Can you work these out from the model? Positions are in its coordinate system, mm. Face numbers are marked on the shaded views. A direction names the side the tool comes from. Round coordinates to 2 decimals unless told otherwise and drop trailing zeros. Write each loop counter-clockwise with the first axis right and the second up, starting at its lowest first coordinate (ties: lowest second). Pieces come first, ordered by that corner, then holes. Notation, with made-up numbers: M 35,56.25 L 73,56.25 A16 ccw 73,84.25 Z; hole C 0.5,76.5 d6. An arc over 180 degrees is marked long. Answer as a JSON object with one key per item and string values. Group by question number.
1) Suppose I cut it at D-D, the plane x = 7. Write out the boundary of the cut face in (y, z), and give its area (3 significant figures).
2) Please list where these lines run through material, in increasing order: L1, parallel to X at y = -2.75, z = 232; L2, parallel to Z at x = 0, y = -4; L3, parallel to Z at x = 11, y = -3.5. Write a range as [from, to].
3) Suppose I cut it at B-B, the plane z = 46.5. Write out the boundary of the cut face in (x, y).
4) Suppose I cut it at C-C, the plane x = -6. Write out the boundary of the cut face in (y, z).
5) Suppose I cut it at A-A, the plane y = 0. Write out the boundary of the cut face in (x, z), and give its area (3 significant figures).
6) I'm going to push flat-ended pins straight in: pin 1 Ø3 at (x, z) = (4.5, 138) entering from +Y; pin 2 Ø6 at (x, z) = (2.5, 237.5) entering from -Y; pin 3 Ø2 at (x, z) = (-5.5, 31.5) entering from +Y; pin 4 Ø10 at (x, y) = (11, 3) entering from -Z. Where does each tip first touch, or does it pass through?
7) On a 3-axis mill with a long thin cutter (end or side, diameter ignored), from which of +Z, -Z, +X, -X, +Y, -Y can I reach the whole of each face in a straight line? I mean the marked faces 1 and 2. Say none if no direction works.
from build123d import *

# Parameters (mm, degrees)
F0_R     = 10.85
F1_DEPTH = 225
F4_DEPTH = 15.21
F6_D     = 2.5
F6_DEPTH = 15
F6_TIP   = 0.7510757738


with BuildPart() as f1:
    # F0 (on Top) → F1 (new body)
    with BuildSketch(Plane.XY):
        Circle(F0_R)
    extrude(amount=F1_DEPTH)

    # F3 (on face) → F4 (join, symmetric)
    with BuildSketch(Plane.YZ):
        Polygon((-10.8373243377, 245), (-10.8373243377, 225), (10.8499713242, 225), align=None)
        Polygon((10.8499713242, 245), (-10.8373243377, 245), (10.8499713242, 225), align=None)
    extrude(amount=F4_DEPTH, both=True)

    # F6
    with Locations(Plane.XZ.offset(10.8373243377)):
        with Locations((11, 232), (0, 232), (-11, 232), (0, 240)):
            Hole(F6_D / 2, depth=F6_DEPTH)
            with Locations((0, 0, -(F6_DEPTH + F6_TIP / 2))):  # 118° drill point
                Cone(0, F6_D / 2, F6_TIP, mode=Mode.SUBTRACT)


solid = f1.part
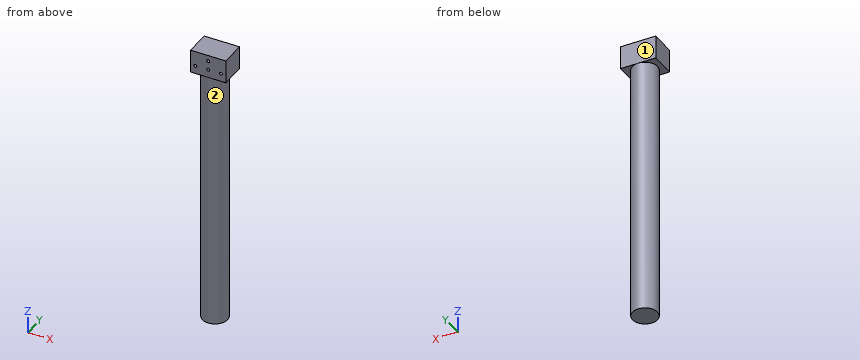
Results:
{
 "1": {"outline": "M -10.84,225 L -8.29,225 L -8.29,0 L 8.29,0 L 8.29,225 L 10.85,225 L 10.85,245 L -10.84,245 Z", "area": "4,160 mm^2"},
 "2": {"L1": "[-15.21, -12.25], [-9.75, -1.25], [1.25, 9.75], [12.25, 15.21]", "L2": "[0, 230.75], [233.25, 238.75], [241.25, 245]", "L3": "[225, 230.75], [233.25, 245]"},
 "3": {"outline": "C 0,0 d21.7"},
 "4": {"outline": "M -10.84,225 L -9.04,225 L -9.04,0 L 9.04,0 L 9.04,225 L 10.85,225 L 10.85,245 L -10.84,245 Z"},
 "5": {"outline": "M -15.21,225 L -10.85,225 L -10.85,0 L 10.85,0 L 10.85,225 L 15.21,225 L 15.21,245 L -15.21,245 Z; hole C -11,232 d2.5; hole C 0,232 d2.5; hole C 0,240 d2.5; hole C 11,232 d2.5", "area": "5,470 mm^2"},
 "6": {"pin 1": "y = 10.43", "pin 2": "y = -10.84", "pin 3": "y = 9.87", "pin 4": "z = 0"},
 "7": {"face 1": "+Z, -Z, +X, -X, +Y", "face 2": "-Z"}
}
